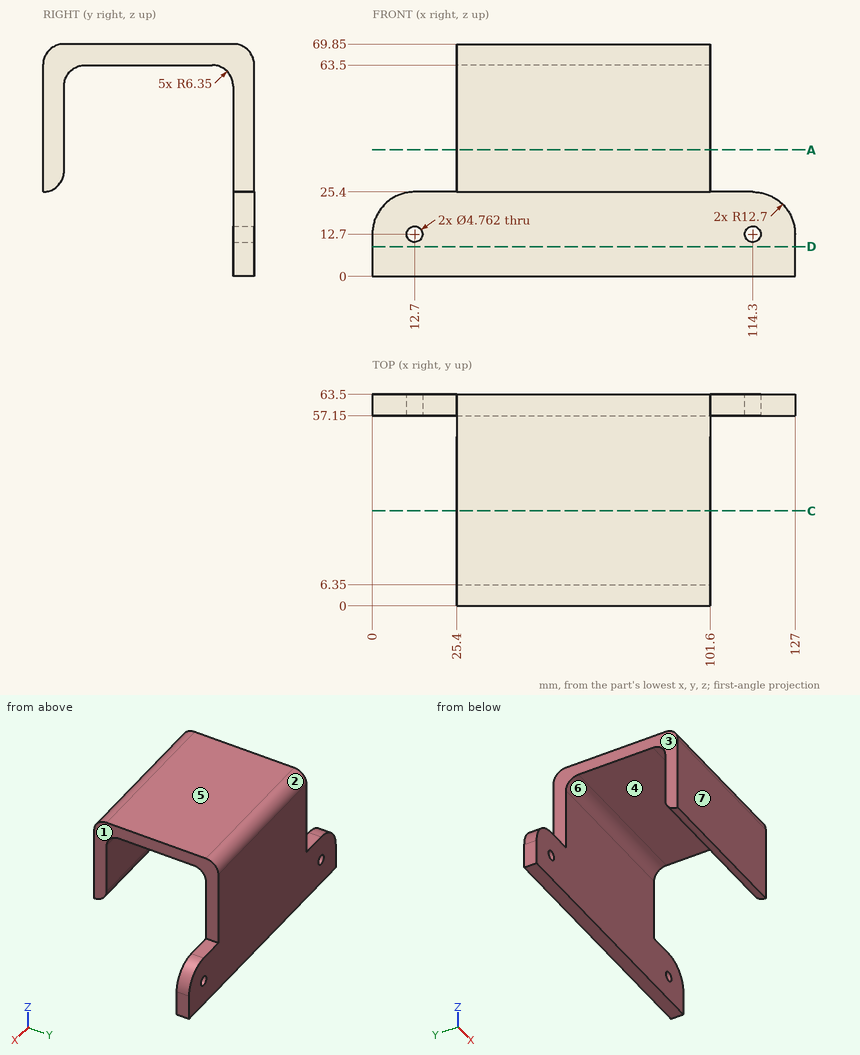
Study the drawing (mm; zero at the part's minimum x, y, z) and answer. A direction names the side the tool comes from. Round coordinates to 2 decimals unless told otherwise and drop trailing zeros. Write each loop counter-clockwise with the first axis right and the second up, starting at its lowest first coordinate (ties: lowest second). Pieces come first, ordered by that corner, then holes. Notation, with made-up numbers: (48.5, 67.5) - (72.5, 67.5) arc R22 ccw to (72.5, 102.5) - close; hole circle Ø11 at (41.25, -24.5). An arc over 180 degrees is marked (long way). Use CSV: the item, a comma, the result in double quotes.
Q1. Each of these flat-tipped pins is pushed along its axis until it touches: pin 1 Ø3 at (x, y) = (18.5, 60.5) entering from +Z; pin 2 Ø4 at (x, y) = (81.5, 11.5) entering from -Z (1 decimal); pin 3 Ø1 at (x, y) = (89.5, 7.5) entering from -Z; pin 4 Ø3 at (x, z) = (114.3, 12.7) entering from +Y. Where does it stop, or does it pass through?
Values:
pin 1,"stops at z = 25.4"
pin 2,"stops at z = 62.6"
pin 3,"stops at z = 59.95"
pin 4,"passes through"
Q2. Find section D-D, the plane z = 9. Write down the section's boundary in (x, y).
Values:
outline,"(0, 57.15) - (127, 57.15) - (127, 63.5) - (0, 63.5) - close"
Q3. Find section C-C, the plane y = 28.5. Write down the section's boundary in (x, z).
Values:
outline,"(25.4, 63.5) - (101.6, 63.5) - (101.6, 69.85) - (25.4, 69.85) - close"
Q4. Straight lines are drawn through the part: line 1 along Z through (x, y) = (12.7, 62); line 2 along Y through (x, z) = (81, 48); line 3 along X through (y, z) = (44, 66). For each, find the intervals that lie inside material, in ascending order.
Values:
line 1,"z = 0 to 10.32, 15.08 to 25.4"
line 2,"y = 0 to 6.35, 57.15 to 63.5"
line 3,"x = 25.4 to 101.6"
Q5. Determine the mould class of the marked faces 5, 6 and 7 for opening direction Y: +Y half, -Y half, draft (parallel to the pull), parting line (faces both ways), or undercut.
Values:
face 5,"draft"
face 6,"undercut"
face 7,"-Y half"
Q6. A tool of negligible diameter and unlimited length cuts with its end or side. For the marked faces 1, 2, 3 and 4, from which of +Z, -Z, +X, -X, +Y, -Y can it reach the whole face along a straight path? Write none if from no direction.
Values:
face 1,"+Z, +X, +Y, -Y"
face 2,"+Z, +X, -X, +Y"
face 3,"+Z, -X, +Y, -Y"
face 4,"-Z, +X, -X"
Q7. Find section A-A, the plane z = 38. Write down the section's boundary in (x, y).
Values:
outline,"(25.4, 0) - (101.6, 0) - (101.6, 6.35) - (25.4, 6.35) - close; (25.4, 57.15) - (101.6, 57.15) - (101.6, 63.5) - (25.4, 63.5) - close"
